```python
from build123d import *

# Parameters (mm, degrees)
SKETCH_1_W          = 500
SKETCH_1_H          = 300
EXTRUDE_1_DEPTH     = 20
SKETCH_2_W          = 450
SKETCH_2_H          = 250
EXTRUDE_2_DEPTH     = 10
SKETCH_3_W          = 400
SKETCH_3_H          = 200
CUT_EXTRUDE_1_DEPTH = 293.232783924
SKETCH_4_W          = 50
SKETCH_4_H          = 150
EXTRUDE_3_DEPTH     = 100


with BuildPart() as part:
    # 草图1 → 凸台-拉伸1 (new body)
    with BuildSketch(Plane.XY):
        Rectangle(SKETCH_1_W, SKETCH_1_H)
    extrude(amount=EXTRUDE_1_DEPTH)

    # 草图2 → 凸台-拉伸2 (add)
    with BuildSketch(Plane.XY):
        Rectangle(SKETCH_2_W, SKETCH_2_H)
    extrude(amount=EXTRUDE_2_DEPTH)

    # 草图3 → 切除-拉伸1 (cut, through all)
    with BuildSketch(Plane.XY):
        Rectangle(SKETCH_3_W, SKETCH_3_H)
    extrude(amount=CUT_EXTRUDE_1_DEPTH, mode=Mode.SUBTRACT)

    # 草图4 → 凸台-拉伸3 (add)
    with BuildSketch(Plane.XY):
        with Locations((0, -200)):
            Rectangle(SKETCH_4_W, SKETCH_4_H)
    extrude(amount=EXTRUDE_3_DEPTH)


solid = part.part
```
Here's how the part is built. I have some questions about the finished solid (model axes, mm). A direction names the side the tool comes from. Give positions to 0.01 mm unless a question says otherwise; leave off trailing zeros. Loops run counter-clockwise (first coordinate to the right, second up) from the corner with the lowest first, then second, coordinate; pieces in that order, holes last. Notation, with made-up numbers: M 38.25,68 L 63.25,68 A37 ccw 63.25,107 Z; hole C 44.25,37 d9. An arc over 180 degrees is marked long. Return JSON: item names as keys, results as strings.
Item 1: Imagine slicing it at B-B on x = 151. List the corners of the cut face in (y, z) for me.
A:
{"outline": "M -150,0 L -100,0 L -100,20 L -150,20 Z; M 100,0 L 150,0 L 150,20 L 100,20 Z"}
Item 2: I'm going to push flat-ended pins straight in: pin 1 Ø16 at (x, z) = (-118, 9.5) entering from -Y; pin 2 Ø15 at (x, z) = (-11.5, 56) entering from +Y; pin 3 Ø12 at (y, z) = (-136.5, 64) entering from +X. Where does each tip first touch, or does it pass through?
A:
{"pin 1": "stops at y = -150", "pin 2": "stops at y = -125", "pin 3": "stops at x = 25"}
Item 3: Imagine slicing it at C-C on x = 13. List the corners of the cut face in (y, z) for me.
A:
{"outline": "M -275,0 L -100,0 L -100,20 L -125,20 L -125,100 L -275,100 Z; M 100,0 L 150,0 L 150,20 L 100,20 Z"}
Item 4: Thinking about a two-plate mould opening in Y: for faces 1 (the flat face through (250, -2, 10)), 2 (the flat face through (-200, -1, 10)), 3 (the flat face through (0, -275, 49)), which applies, released by +Y, released by -Y, zero draft, split by the parting line, or undercut?
A:
{"face 1": "zero draft", "face 2": "undercut", "face 3": "released by -Y"}
Item 5: Please list where these lines run through material, in increasing order: line 1 (Y direction, x = -173.5, z = 6.5); line 2 (X direction, y = 71, z = 18); line 3 (X direction, y = -169, z = 92).
A:
{"line 1": "y = -150 to -100, 100 to 150", "line 2": "x = -250 to -200, 200 to 250", "line 3": "x = -25 to 25"}
Item 6: Imagine slicing it at A-A on y = -60. List the corners of the cut face in (x, z) for me, then the cut area to 3 significant figures.
A:
{"outline": "M -250,0 L -200,0 L -200,20 L -250,20 Z; M 200,0 L 250,0 L 250,20 L 200,20 Z", "area": "2,000 mm^2"}
Item 7: Imagine slicing it at D-D on z = 69.5. List the corners of the cut face in (x, y) for me.
A:
{"outline": "M -25,-275 L 25,-275 L 25,-125 L -25,-125 Z"}
Item 8: On a 3-axis mill with a long thin cutter (end or side, diameter ignored), from which of +Z, -Z, +X, -X, +Y, -Y can I reach the whole of each face in a straight line? I mean faces 4 (the flat face through (0, -125, 59)), 5 (the flat face through (136, -150, 10)), 6 (the flat face through (-139, -150, 10)), 7 (the flat face through (-3, -100, 10)). Say none if no direction works.
A:
{"face 4": "+Z, +X, -X, +Y", "face 5": "+Z, -Z, +X, -Y", "face 6": "+Z, -Z, -X, -Y", "face 7": "+Z, -Z"}
